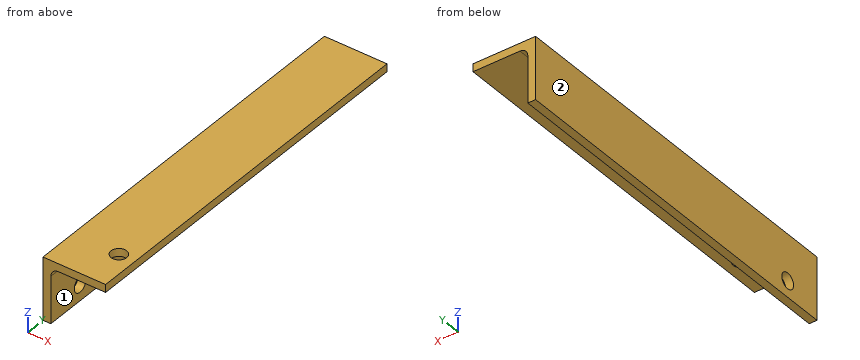
```python
from build123d import *

# Parameters (mm, degrees)
BOSS_EXTRUDE1_DEPTH = 152.4
FILLET2_R           = 3.175
SKETCH3_R           = 3.175
CUT_EXTRUDE2_DEPTH  = 157.576115675
CUT_EXTRUDE3_REACH  = 158.576
SKETCH4_R           = 3.175


with BuildPart() as part:
    # Sketch1 → Boss-Extrude1 (new body)
    with BuildSketch(Plane(origin=(0, 0, 0), x_dir=(1, 0, 0), z_dir=(0, 1, 0))):
        Polygon((0, 0), (0, -25.4), (25.4, -25.4), (25.4, -22.225), (3.175, -22.225), (3.175, 0), align=None)
    extrude(amount=BOSS_EXTRUDE1_DEPTH)

    # Fillet2
    fillet2_edges = [part.edges().sort_by_distance(p)[0] for p in [
        (3.175, 76.2, 22.225),
    ]]
    fillet(fillet2_edges, radius=FILLET2_R)

    # Sketch3 → Cut-Extrude2 (cut, through all)
    with BuildSketch(Plane.ZY):
        with Locations((6.604, 15.875)):
            Circle(SKETCH3_R)
    extrude(amount=-CUT_EXTRUDE2_DEPTH, mode=Mode.SUBTRACT)

    # Sketch4 → Cut-Extrude3 (cut, up to next)
    with BuildSketch(Plane.XY.offset(25.4), mode=Mode.PRIVATE) as cut_extrude3_sk1:
        with Locations((18.796, 16.002)):
            Circle(SKETCH4_R)
    cut_extrude3_tool1 = extrude(cut_extrude3_sk1.sketch, amount=-CUT_EXTRUDE3_REACH, mode=Mode.PRIVATE) & part.part
    add(cut_extrude3_tool1.solids().sort_by_distance((18.796, 16.002, 25.4))[0], mode=Mode.SUBTRACT)


solid = part.part
```
Verification items for the finished model (mm, model axes). Face numbers are marked on the shaded views. A direction names the side the tool comes from. Coordinates: 2 decimals unless noted, no trailing zeros. Loops run counter-clockwise (first coordinate to the right, second up) from the corner with the lowest first, then second, coordinate; pieces in that order, holes last. Notation, with made-up numbers: (73, -15.75) - (97, -15.75) arc R26 ccw to (97, 6.25) - close; hole circle Ø9 at (16, 24.25). An arc over 180 degrees is marked (long way). Answer as a JSON object with one key per item and string values.
(1) Cross-section at B-B, the plane z = 8.5. Record the boundary of the cut face in (x, y) (3 decimals), then the cut area to 3 significant figures.
Response:
{"outline": "(0, 0) - (3.175, 0) - (3.175, 13.328) - (0, 13.328) - close; (0, 18.422) - (3.175, 18.422) - (3.175, 152.4) - (0, 152.4) - close", "area": "468 mm²"}
(2) Cross-section at D-D, the plane z = 16.25. Record the boundary of the cut face in (x, y) (3 decimals), then the cut area to 3 significant figures.
Response:
{"outline": "(0, 0) - (3.175, 0) - (3.175, 152.4) - (0, 152.4) - close", "area": "484 mm²"}
(3) Cross-section at A-A, the plane x = 17.5. Record the boundary of the cut face in (y, z) (3 decimals).
Response:
{"outline": "(0, 22.225) - (13.104, 22.225) - (13.104, 25.4) - (0, 25.4) - close; (18.9, 22.225) - (152.4, 22.225) - (152.4, 25.4) - (18.9, 25.4) - close"}
(4) Cross-section at C-C, the plane y = 114.5. Record the boundary of the cut face in (x, z) (3 decimals).
Response:
{"outline": "(0, 0) - (3.175, 0) - (3.175, 19.05) arc R3.175 cw to (6.35, 22.225) - (25.4, 22.225) - (25.4, 25.4) - (0, 25.4) - close"}
(5) Go/stop test with flat-tipped pins: pin 1 Ø2 at (y, z) = (37.5, 12.5) entering from +X (3 decimals); pin 2 Ø1 at (x, y) = (14, 52) entering from -Z (3 decimals). Record where each tip stops, or that it passes through.
Response:
{"pin 1": "stops at x = 3.175", "pin 2": "stops at z = 22.225"}
(6) Access from +Z, -Z, +X, -X, +Y, -Y to the whole of each face (thin tool, end or side, straight path). Record for the marked faces 1 and 2.
Response:
{"face 1": "-Z, +X, +Y, -Y", "face 2": "+Z, -Z, -X, +Y, -Y"}
(7) Scan lines: line 1 along Z through (x, y) = (14.75, 80.5) (3 decimals); line 2 along X through (y, z) = (145, 16) (3 decimals); line 3 along X through (y, z) = (77, 21). Record each from-to range of solid material in increasing order.
Response:
{"line 1": "z = 22.225 to 25.4", "line 2": "x = 0 to 3.175", "line 3": "x = 0 to 3.84"}
